Check sheet for the modelled part. Datum: model origin and axes. Units: mm. A direction names the side the tool comes from. Give positions to 0.01 mm unless a question says otherwise; leave off trailing zeros. Order: outer loops, then holes, each group sorted by start corner. A loop starts at its lowest first (then second) coordinate and runs counter-clockwise, first axis right, second up. Notation, with made-up numbers: (44.5, 77.5) -> (78.5, 77.5) arc R10 cw to (78.5, 87.5) -> close; hole circle Ø3 at (50, 68). An arc over 180 degrees is marked (long way). Answer in a Markdown table with one row per item. Add a question column.
(1) Cross-section at A-A (y = 40). Record the cut outline in (x, z), then the cut area to 3 significant figures.
(2) Cross-section at D-D (x = 14). Record the cut outline in (y, z), then the cut area to 3 significant figures.
(3) Set-up check for faces 5 (the face through (5, 35, 0)), 6 (the face through (3, -31, -5)), 7 (the face through (3, -31, 5)), 8 (the face through (-5, 32, 0)), 9 (the face through (-35, -23, 0)): record each of +Z, -Z, +X, -X, +Y, -Y from which the full face is reachable in a straight line by a thin tool's end or side.
(4) Go/stop test with flat-tipped pins: pin 1 (3 mm diameter, centred on y = 40, z = 0, fed in from -X); pin 2 (3 mm diameter, centred on x = -7.5, z = -1.5, fed in from +Y); pin 3 (4 mm diameter, centred on x = 5.5, y = 24, fed in from -Z); pin 4 (10 mm diameter, centred on y = 39, z = -2.5, fed in from -X). Record where each tip stops, or that it passes through.
(5) Release check for a two-part mould opening along Y. For faces 1 (the face through (14.72, 6.43, 0.07)), 2 (the face through (0, 50, 0)), 3 (the face through (-40, -15, 0)), 4 (the face through (0, -30, 0)) record: released by +Y, released by -Y, zero draft, split by the parting line, or undercut.
(6) Cross-section at C-C (x = -2.5). Record the cut outline in (y, z).
(7) Thickness scan on L1, parallel to X at y = -24, z = -3.25; L2, parallel to Y at x = 36.5, z = -0.25; L3, parallel to X at y = 39, z = -3. Record the ranges inside material, lowest first. Write a range as [from, to].
(8) Cross-section at B-B (z = 0). Record the cut outline in (x, y).
```python
from build123d import *

# Parameters (mm, degrees)
F1_DEPTH = 5
F2_R     = 2.5
F3_DEPTH = 5


with BuildPart() as f1:
    # F0 (on Top) → F1 (new body, symmetric)
    with BuildSketch(Plane.XY):
        Polygon((-45, -40), (0, -40), (45, -40), (45, 0), (45, 7.320508), (5, 20), (5, 31.33975), (-5, 31.33975), (-5, 12.679492), (35, 0), (35, -30), (-35, -30), (-35, -15), (-45, -15), align=None)
    extrude(amount=F1_DEPTH, both=True)

    # F2 (on Right) → F3 (join, symmetric)
    with BuildSketch(Plane.YZ):
        with BuildLine():
            Line((31.339746, 5), (31.339746, -5))
            ThreePointArc((31.339746, -5), (50, 0), (31.339746, 5))
        make_face()
        with Locations((40, 0)):
            Circle(F2_R, mode=Mode.SUBTRACT)
    extrude(amount=F3_DEPTH, both=True)


solid = f1.part
```
Answer below:
| question | item | result |
|---|---|---|
| 1 | outline | (-5, -10) -> (5, -10) -> (5, -2.5) -> (-5, -2.5) -> close; (-5, 2.5) -> (5, 2.5) -> (5, 10) -> (-5, 10) -> close |
| 1 | area | 150 mm² |
| 2 | outline | (-40, -5) -> (-30, -5) -> (-30, 5) -> (-40, 5) -> close; (6.66, -5) -> (17.15, -5) -> (17.15, 5) -> (6.66, 5) -> close |
| 2 | area | 205 mm² |
| 3 | face 5 | +Z, -Z, +X, +Y |
| 3 | face 6 | -Z, +X, -X, -Y |
| 3 | face 7 | +Z, +X, -X, -Y |
| 3 | face 8 | +Z, -Z, -X, +Y |
| 3 | face 9 | +Z, -Z, +Y |
| 4 | pin 1 | passes through |
| 4 | pin 2 | stops at y = -30 |
| 4 | pin 3 | stops at z = -5 |
| 4 | pin 4 | stops at x = -5 |
| 5 | face 1 | undercut |
| 5 | face 2 | split by the parting line |
| 5 | face 3 | released by +Y |
| 5 | face 4 | undercut |
| 6 | outline | (-40, -5) -> (-30, -5) -> (-30, 5) -> (-40, 5) -> close; (11.89, -5) -> (31.34, -5) arc R10 ccw (long way) to (31.34, 5) -> (11.89, 5) -> close; hole circle Ø5 at (40, 0) |
| 7 | L1 | x = [-45, -35], [35, 45] |
| 7 | L2 | y = [-40, 10.01] |
| 7 | L3 | x = [-5, 5] |
| 8 | outline | (-45, -40) -> (45, -40) -> (45, 7.32) -> (5, 20) -> (5, 37.5) -> (-5, 37.5) -> (-5, 12.68) -> (35, 0) -> (35, -30) -> (-35, -30) -> (-35, -15) -> (-45, -15) -> close; (-5, 42.5) -> (5, 42.5) -> (5, 50) -> (-5, 50) -> close |
